Could you check a few things on this model? Use its own coordinates, in mm. Face numbers are marked on the shaded views. Round coordinates to 2 decimals unless told otherwise and drop trailing zeros. Order: outer loops, then holes, each group sorted by start corner. A loop starts at its lowest first (then second) coordinate and runs counter-clockwise, first axis right, second up.
```python
from build123d import *

# Parameters (mm, degrees)
F0_R     = 1.905
F1_DEPTH = 3.175
F2_DEPTH = 3.175
F3_DEPTH = 12.7
F5_DEPTH = 9.525
F6_R     = 6.35
F9_DEPTH = 44.45


with BuildPart() as f1:
    # F0 (on Top) → F1 (new body)
    with BuildSketch(Plane.XY):
        with BuildLine():
            Line((2.1997045256, 3.81), (-0.1821025232, 7.9354108224))
            ThreePointArc((-0.1821025232, 7.9354108224), (-6.8740766425, -3.96875), (6.7812161001, -4.1254108224))
            Line((6.7812161001, -4.1254108224), (4.3994090512, 0))
            Line((4.3994090512, 0), (2.1997045256, -3.81))
            Line((2.1997045256, -3.81), (-2.1997045256, -3.81))
            Line((-2.1997045256, -3.81), (-4.3994090512, 0))
            Line((-4.3994090512, 0), (-2.1997045256, 3.81))
            Line((-2.1997045256, 3.81), (2.1997045256, 3.81))
        make_face()
        with BuildLine():
            ThreePointArc((4.1641356391, 6.7575055034), (2.0762977072, 7.6611287733), (-0.1821025232, 7.9354108224))
            Line((-0.1821025232, 7.9354108224), (2.1997045256, 3.81))
            Line((2.1997045256, 3.81), (4.3994090512, 0))
            Line((4.3994090512, 0), (6.7812161001, -4.1254108224))
            ThreePointArc((6.7812161001, -4.1254108224), (7.672880993, -2.0324378264), (7.9342392518, 0.2274944966))
            Line((7.9342392518, 0.2274944966), (4.1641356391, 6.7575055034))
        make_face()
        Polygon((4.3994090512, 0), (2.1997045256, 3.81), (-2.1997045256, 3.81), (-4.3994090512, 0), (-2.1997045256, -3.81), (2.1997045256, -3.81), align=None)
        Circle(F0_R, mode=Mode.SUBTRACT)
    extrude(amount=-F1_DEPTH)

    # F0 (on Top) → F2 (join)
    with BuildSketch(Plane.XY):
        with BuildLine():
            Line((-1.0837612628, 9.4971295705), (-4.4059530098, 15.2513344687))
            ThreePointArc((-4.4059530098, 15.2513344687), (-15.7183103368, -2.2249371126), (0, -15.875))
            ThreePointArc((0, -15.875), (5.9323031071, -14.7249246125), (11.0050665866, -11.4413344687))
            Line((11.0050665866, -11.4413344687), (6.7812161001, -4.1254108224))
            ThreePointArc((6.7812161001, -4.1254108224), (-6.8740766425, -3.96875), (-0.1821025232, 7.9354108224))
            Line((-0.1821025232, 7.9354108224), (-1.0837612628, 9.4971295705))
        make_face()
        Polygon((-12.5754425904, 29.4013054943), (-4.4059530098, 15.2513344687), (-1.0837612628, 9.4971295705), (1.6658693942, 11.0846295705), (-9.8258119334, 30.9888054943), align=None)
        with BuildLine():
            ThreePointArc((0, -15.875), (-15.7183103368, -2.2249371126), (-4.4059530098, 15.2513344687))
            Line((-4.4059530098, 15.2513344687), (-12.5754425904, 29.4013054943))
            Line((-12.5754425904, 29.4013054943), (-15.7504425904, 34.9005668084))
            ThreePointArc((-15.7504425904, 34.9005668084), (-26.8159478457, 3.6374215932), (0, -15.875))
        make_face()
        with BuildLine():
            Line((1.6658693942, 11.0846295705), (-1.0837612628, 9.4971295705))
            Line((-1.0837612628, 9.4971295705), (-0.1821025232, 7.9354108224))
            ThreePointArc((-0.1821025232, 7.9354108224), (2.0762977072, 7.6611287733), (4.1641356391, 6.7575055034))
            Line((4.1641356391, 6.7575055034), (1.6658693942, 11.0846295705))
        make_face()
        Polygon((-15.7504425904, 34.9005668084), (-12.5754425904, 29.4013054943), (-9.8258119334, 30.9888054943), (-13.0008119334, 36.4880668084), align=None)
        with BuildLine():
            Line((6.7812161001, -4.1254108224), (11.0050665866, -11.4413344687))
            ThreePointArc((11.0050665866, -11.4413344687), (12.1601025371, -10.2052697803), (13.1770447672, -8.8533110305))
            Line((13.1770447672, -8.8533110305), (7.9342392518, 0.2274944966))
            ThreePointArc((7.9342392518, 0.2274944966), (7.672880993, -2.0324378264), (6.7812161001, -4.1254108224))
        make_face()
        with BuildLine():
            ThreePointArc((4.1641356391, 6.7575055034), (2.0762977072, 7.6611287733), (-0.1821025232, 7.9354108224))
            Line((-0.1821025232, 7.9354108224), (2.1997045256, 3.81))
            Line((2.1997045256, 3.81), (4.3994090512, 0))
            Line((4.3994090512, 0), (6.7812161001, -4.1254108224))
            ThreePointArc((6.7812161001, -4.1254108224), (7.672880993, -2.0324378264), (7.9342392518, 0.2274944966))
            Line((7.9342392518, 0.2274944966), (4.1641356391, 6.7575055034))
        make_face()
        with BuildLine():
            Line((2.1997045256, 3.81), (-0.1821025232, 7.9354108224))
            ThreePointArc((-0.1821025232, 7.9354108224), (-6.8740766425, -3.96875), (6.7812161001, -4.1254108224))
            Line((6.7812161001, -4.1254108224), (4.3994090512, 0))
            Line((4.3994090512, 0), (2.1997045256, -3.81))
            Line((2.1997045256, -3.81), (-2.1997045256, -3.81))
            Line((-2.1997045256, -3.81), (-4.3994090512, 0))
            Line((-4.3994090512, 0), (-2.1997045256, 3.81))
            Line((-2.1997045256, 3.81), (2.1997045256, 3.81))
        make_face()
    extrude(amount=F2_DEPTH)

    # F0 (on Top) → F3 (join)
    with BuildSketch(Plane.XY):
        with BuildLine():
            Line((6.7812161001, -4.1254108224), (11.0050665866, -11.4413344687))
            ThreePointArc((11.0050665866, -11.4413344687), (12.1601025371, -10.2052697803), (13.1770447672, -8.8533110305))
            Line((13.1770447672, -8.8533110305), (7.9342392518, 0.2274944966))
            ThreePointArc((7.9342392518, 0.2274944966), (7.672880993, -2.0324378264), (6.7812161001, -4.1254108224))
        make_face()
        with BuildLine():
            Line((1.6658693942, 11.0846295705), (-1.0837612628, 9.4971295705))
            Line((-1.0837612628, 9.4971295705), (-0.1821025232, 7.9354108224))
            ThreePointArc((-0.1821025232, 7.9354108224), (2.0762977072, 7.6611287733), (4.1641356391, 6.7575055034))
            Line((4.1641356391, 6.7575055034), (1.6658693942, 11.0846295705))
        make_face()
        Polygon((-12.5754425904, 29.4013054943), (-4.4059530098, 15.2513344687), (-1.0837612628, 9.4971295705), (1.6658693942, 11.0846295705), (-9.8258119334, 30.9888054943), align=None)
        Polygon((-15.7504425904, 34.9005668084), (-12.5754425904, 29.4013054943), (-9.8258119334, 30.9888054943), (-13.0008119334, 36.4880668084), align=None)
    extrude(amount=F3_DEPTH)

    # F4 (on face) → F5 (join)
    with BuildSketch(Plane.XY.offset(3.175)):
        with BuildLine():
            Line((4.3994090512, 0), (6.7812161001, -4.1254108224))
            ThreePointArc((6.7812161001, -4.1254108224), (7.672880993, -2.0324378264), (7.9342392518, 0.2274944966))
            Line((7.9342392518, 0.2274944966), (4.1641356391, 6.7575055034))
            ThreePointArc((4.1641356391, 6.7575055034), (2.0762977072, 7.6611287733), (-0.1821025232, 7.9354108224))
            Line((-0.1821025232, 7.9354108224), (2.1997045256, 3.81))
            Line((2.1997045256, 3.81), (4.3994090512, 0))
        make_face()
    extrude(amount=F5_DEPTH)

    # F6
    f6_edges = [f1.edges().sort_by_distance(p)[0] for p in [
        (-14.375627, 35.694317, 12.7),
        (12.160103, -10.20527, 12.7),
    ]]
    fillet(f6_edges, radius=F6_R)


with BuildPart() as f8_1:
    # F8: instance of F1
    add(f1.part.mirror(Plane(origin=(-0.1702882742, -0.0983159809, -22.225), x_dir=(1, 0, 0), z_dir=(0, 0, -1))))


with BuildPart() as f1_1:
    add(f1.part)

    add(f8_1.part)  # F9 merges F8_1
    # F0 (on Top) → F9 (join, through all)
    with BuildSketch(Plane.XY):
        Polygon((-15.7504425904, 34.9005668084), (-12.5754425904, 29.4013054943), (-9.8258119334, 30.9888054943), (-13.0008119334, 36.4880668084), align=None)
    extrude(amount=-F9_DEPTH)


solid = f1_1.part
```
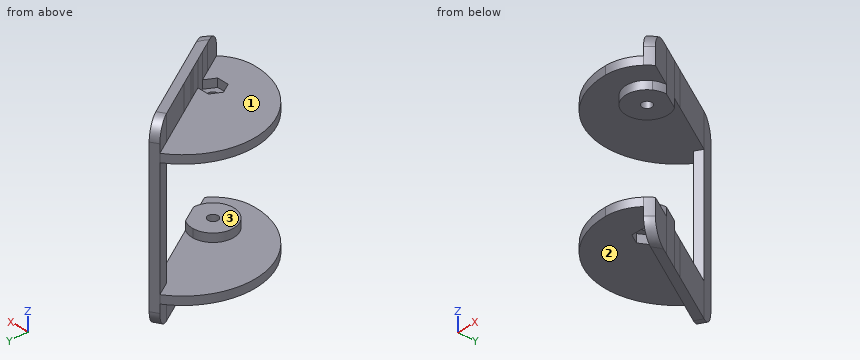
Q1. Imagine slicing it at B-B, the plane x = -17. Please give me the cut outline in (y, z) (3 decimals).
Q2. Imagine slicing it at D-D, the plane x = -9. Please give me the cut outline in (y, z) (3 decimals), then the cut area to 3 significant figures.
Q3. We'd pull the mould along Z, two halves only. Please class the marked faces 1, 2 and 3: released by +Z, released by -Z, zero draft, split by the parting line, or undercut.
Q4. For P1, Ø1, axis at x = -1, z = 2.5, coming from the -Y side; P2, Ø1.6, axis at x = -0.5, z = -45.5, coming from the +Y side; P3, Ø6, axis at x = -21.5, y = 13, coming from the +Z side (3 decimals); P4, Ø4, axis at x = -7, z = -10, coming from the -Y side, each with a flat end and sliding along its axis, tell me the tip position at first contact or that it passes through.
Q5. I need wall thicknesses on L1, parallel to Y at x = 0, z = -1 (1 decimal); L2, parallel to Z at x = -11, y = -3 (3 decimals); L3, parallel to Z at x = -6.5, y = 19.5. Which ranges of each line are inside material? Lowest first, please.
Q6. Imagine slicing it at C-C, the plane y = 28. Please give me the cut outline in (x, z) (3 decimals), then the cut area to 3 significant figures.
Filled in:
1. outline: (-10.308, -47.625) - (34.014, -47.625) - (34.014, -44.45) - (-10.308, -44.45) - close; (-10.308, 0) - (34.014, 0) - (34.014, 3.175) - (-10.308, 3.175) - close
2. outline: (-14.487, -47.625) - (23.208, -47.625) - (23.208, -57.15) - (29.558, -57.15) - (29.558, -44.45) - (-14.487, -44.45) - close; (-14.487, 0) - (29.558, 0) - (29.558, 12.7) - (23.208, 12.7) - (23.208, 3.175) - (-14.487, 3.175) - close
2. area: 401 mm2
3. face 1: released by +Z
3. face 2: released by -Z
3. face 3: undercut
4. P1: stops at y = -15.88
4. P2: stops at y = 16.22
4. P3: stops at z = 3.175
4. P4: passes through
5. L1: y = -7.9 to -1.9, 1.9 to 7.9
5. L2: z = -47.625 to -44.45, 0 to 3.175
5. L3: z = -57.15 to -44.45, 0 to 12.7
6. outline: (-22.875, -47.625) - (-11.766, -47.625) - (-11.766, -57.15) - (-8.1, -57.15) - (-8.1, -44.45) - (-22.875, -44.45) - close; (-22.875, 0) - (-8.1, 0) - (-8.1, 12.7) - (-11.766, 12.7) - (-11.766, 3.175) - (-22.875, 3.175) - close
6. area: 164 mm2
